from build123d import *

# Parameters (mm, degrees)
SKETCH002_W     = 30
SKETCH002_H     = 30
PAD002_DEPTH    = 20
CHAMFER_SIZE    = 1
PAD003_DEPTH    = 15
SKETCH004_W     = 10
SKETCH004_H     = 20
POCKET_DEPTH    = 35
CHAMFER001_SIZE = 16
SKETCH005_R     = 2.25
POCKET001_DEPTH = 5.001
PAD004_DEPTH    = 2
CHAMFER002_SIZE = 4
SKETCH017_R     = 2
POCKET004_DEPTH = 30.001
PAD011_DEPTH    = 3


with BuildPart() as part:
    # Sketch002 → Pad002 (new body, symmetric)
    with BuildSketch(Plane.XY):
        Rectangle(SKETCH002_W, SKETCH002_H)
        Polygon((10.05, 3.05), (7.05, 3.05), (7.05, -3.05), (10.05, -3.05), (10.05, -10.05), (3.05, -10.05), (3.05, -7.05), (-3.05, -7.05), (-3.05, -10.05), (-10.05, -10.05), (-10.05, -3.05), (-7.05, -3.05), (-7.05, 3.05), (-10.05, 3.05), (-10.05, 10.05), (-3.05, 10.05), (-3.05, 7.05), (3.05, 7.05), (3.05, 10.05), (10.05, 10.05), align=None, mode=Mode.SUBTRACT)
    extrude(amount=PAD002_DEPTH, both=True)

    # Chamfer
    chamfer_edges = [part.edges().sort_by_distance(p)[0] for p in [
        (-10.05, 3.05, 0),
        (-3.05, 10.05, 0),
        (-10.05, -3.05, 0),
        (-3.05, -10.05, 0),
        (3.05, -10.05, 0),
        (10.05, -3.05, 0),
        (10.05, 3.05, 0),
        (3.05, 10.05, 0),
    ]]
    chamfer(chamfer_edges, length=CHAMFER_SIZE)

    # Sketch003 → Pad003 (join, symmetric)
    with BuildSketch(Plane.YZ):
        Polygon((-15, -20), (-40.05, -20), (-65.05, -20), (-65.05, 0), (-45.05, 20), (-15, 20), align=None)
    extrude(amount=PAD003_DEPTH, both=True)

    # Sketch004 (on Face35 of Pad003) → Pocket (cut)
    with BuildSketch(Plane.XY.offset(20)):
        with Locations((0, -51.05)):
            Rectangle(SKETCH004_W, SKETCH004_H)
    extrude(amount=-POCKET_DEPTH, mode=Mode.SUBTRACT)

    # Chamfer001
    chamfer001_edges = [part.edges().sort_by_distance(p)[0] for p in [
        (0, -41.05, 20),
    ]]
    chamfer(chamfer001_edges, length=CHAMFER001_SIZE)

    # Sketch005 (on Face10 of Chamfer001) → Pocket001 (cut, through all)
    with BuildSketch(Plane.XY.offset(-15)):
        with Locations((0, -46.05)):
            Circle(SKETCH005_R)
        with Locations((0, -56.05)):
            Circle(SKETCH005_R)
    extrude(amount=-POCKET001_DEPTH, mode=Mode.SUBTRACT)

    # Sketch006 → Pad004 (join, symmetric)
    with BuildSketch(Plane.XZ):
        Polygon((16, -20), (20, -20), (20, -8), (15, -3), (15, -13), (17, -13), (15.5, -18), align=None)
    extrude(amount=PAD004_DEPTH, both=True)

    # Chamfer002
    chamfer002_edges = [part.edges().sort_by_distance(p)[0] for p in [
        (-15, -65.05, -10),
        (15, -65.05, -10),
        (-15, 15, 0),
        (15, 15, 0),
    ]]
    chamfer(chamfer002_edges, length=CHAMFER002_SIZE)

    # Sketch017 (on Face9 of Chamfer002) → Pocket004 (cut, through all)
    with BuildSketch(Plane.YZ.offset(15)):
        with Locations((-51.05, 0)):
            Circle(SKETCH017_R)
    extrude(amount=-POCKET004_DEPTH, mode=Mode.SUBTRACT)

    # Sketch019 (on Face12 of Pocket004) → Pad011 (join)
    with BuildSketch(Plane(origin=(0, 0, -20), x_dir=(1, 0, 0), z_dir=(0, 0, -1))):
        Polygon((15, 34.721573), (18, 31.721573), (18, 23.721573), (15, 20.721573), (15, 17.893146), (20, 22.893146), (20, 32.55), (15, 37.55), align=None)
    pad011 = extrude(amount=-PAD011_DEPTH)

    # Mirrored001: Pad011 across Sketch019 V_Axis
    add(pad011.mirror(Plane(origin=(0, 0, -20), x_dir=(0, 0, -1), z_dir=(1, 0, 0))))


solid = part.part
Part model, mm, in its own coordinate system. A direction names the side the tool comes from. Give positions to 0.01 mm unless a question says otherwise; leave off trailing zeros. Order: outer loops, then holes, each group sorted by start corner. A loop starts at its lowest first (then second) coordinate and runs counter-clockwise, first axis right, second up. Notation, with made-up numbers: (30, 7) - (34, 7) arc R8 ccw to (34, 20) - close; hole circle Ø10 at (-33, 54). An arc over 180 degrees is marked (long way). One line per question, with ' | ' between items.
1. Drill centre lines: probe 1 along Y at (x, z) = (0, -18); probe 2 along X at (y, z) = (8, -0.5); probe 3 along Y at (x, z) = (-9, 17). Where is each one in solid material? Low to high.
Filled in:
probe 1: -65.05 to -58.3, -53.8 to -48.3, -43.8 to -7.05, 7.05 to 15 | probe 2: -15 to -10.05, -3.05 to 3.05, 10.05 to 15 | probe 3: -48.05 to -10.05, -3.05 to 3.05, 10.05 to 15
2. Band-saw the part on D-D on x = -14. List the corners of the cut face in (y, z), then the cut area to 3 significant figures.
Filled in:
outline: (-62.05, -20) - (12, -20) - (12, 20) - (-45.05, 20) - (-62.05, 3) - close; hole circle Ø4 at (-51.05, 0) | area: 2,800 mm²
3. Drop flat-ended pins along their axis: P1, Ø1.5, axis at x = 16.5, z = -13.5, coming from the +Y side; P2, Ø1.6, axis at y = -8, z = -3.5, coming from the +X side; P3, Ø1.6, axis at x = -8, z = 4.5, coming from the -Y side. Give the stop position or say it passes through.
Filled in:
P1: y = 2 | P2: x = 15 | P3: y = -61.35
4. Band-saw the part on C-C on y = -51.05. List the corners of the cut face in (x, z).
Filled in:
outline: (-15, -20) - (15, -20) - (15, -2) - (5, -2) - (5, -15) - (-5, -15) - (-5, -2) - (-15, -2) - close; (-15, 2) - (-5, 2) - (-5, 14) - (-15, 14) - close; (5, 2) - (15, 2) - (15, 14) - (5, 14) - close
5. Band-saw the part on A-A on y = 6. List the corners of the cut face in (x, z).
Filled in:
outline: (-15, -20) - (-10.05, -20) - (-10.05, 20) - (-15, 20) - close; (10.05, -20) - (15, -20) - (15, 20) - (10.05, 20) - close
6. Band-saw the part on B-B on x = 0. List the corners of the cut face in (y, z).
Filled in:
outline: (-65.05, -20) - (-58.3, -20) - (-58.3, -15) - (-61.05, -15) - (-61.05, 4) - (-65.05, 0) - close; (-53.8, -20) - (-48.3, -20) - (-48.3, -15) - (-53.8, -15) - close; (-43.8, -20) - (-7.05, -20) - (-7.05, 20) - (-25.05, 20) - (-41.05, 4) - (-41.05, -15) - (-43.8, -15) - close; (7.05, -20) - (15, -20) - (15, 20) - (7.05, 20) - close
7. Pull direction X, two halves, no side cores. Call faces 1 (the face through (0, -15, 20)), 2 (the face through (-17.465, -20.358, -18.521)), 3 (the face through (8, 3.05, 0)): +X half, -X half, draft (parallel to the pull), parting line (faces both ways), or undercut.
Filled in:
face 1: draft | face 2: -X half | face 3: undercut
8. Which spindle directions (+Z, -Z, +X, -X, +Y, -Y) get a long thin tool onto all of the face, cutting with end or side? Do faces 4 (the face through (17, 2, -11)), 5 (the face through (-5, -47, 3)), 6 (the face through (17, -2, -11)), 7 (the face through (0, -7.05, 0)). Say none if no direction does.
Filled in:
face 4: +Z, -Z, +X, +Y | face 5: +Z | face 6: +Z, -Z, +X | face 7: +Z, -Z
